```python
from build123d import *

# Parameters (mm, degrees)
SKETCH1_W           = 70
SKETCH1_H           = 55
BOSS_EXTRUDE1_DEPTH = 2
SKETCH2_W           = 73.35025282
SKETCH2_H           = 59
BOSS_EXTRUDE3_DEPTH = 2
BOSS_EXTRUDE4_DEPTH = 28
BOSS_EXTRUDE5_DEPTH = 34
SKETCH7_W           = 3
SKETCH7_H           = 23
CUT_EXTRUDE1_DEPTH  = 11
SKETCH9_R           = 1.4
CUT_EXTRUDE2_DEPTH  = 11
SKETCH10_W          = 8
SKETCH10_H          = 10
BOSS_EXTRUDE6_DEPTH = 5
CUT_EXTRUDE3_REACH  = 35.573
SKETCH12_W          = 13
SKETCH12_H          = 2
BOSS_EXTRUDE7_DEPTH = 6
SKETCH13_R          = 1.45
CUT_EXTRUDE4_DEPTH  = 10
BOSS_EXTRUDE8_DEPTH = 10
SKETCH15_R          = 1.4
CUT_EXTRUDE5_DEPTH  = 10


with BuildPart() as part:
    # Sketch1 → Boss-Extrude1 (new body)
    with BuildSketch(Plane(origin=(0, 0, 0), x_dir=(1, 0, 0), z_dir=(0, 1, 0))):
        with Locations((35, -27.5)):
            Rectangle(SKETCH1_W, SKETCH1_H)
    extrude(amount=BOSS_EXTRUDE1_DEPTH)

    # Sketch2 → Boss-Extrude3 (add)
    with BuildSketch(Plane(origin=(0, 0, 0), x_dir=(1, 0, 0), z_dir=(0, 1, 0))):
        with Locations((35.32487359, -27.5)):
            Rectangle(SKETCH2_W, SKETCH2_H)
    extrude(amount=BOSS_EXTRUDE3_DEPTH)

    # Sketch3 → Boss-Extrude4 (add)
    with BuildSketch(Plane(origin=(0, 2, 0), x_dir=(1, 0, 0), z_dir=(0, 1, 0))):
        Polygon((-1.35025282, 2), (72, 2), (72, -57), (-1.35025282, -57), (-1.35025282, -55), (70, -55), (70, 0), (-1.35025282, 0), align=None)
    extrude(amount=BOSS_EXTRUDE4_DEPTH)

    # Sketch5 → Boss-Extrude5 (add)
    with BuildSketch(Plane(origin=(0, 2, 0), x_dir=(1, 0, 0), z_dir=(0, 1, 0))):
        Polygon((11.64974718, 0), (8.64974718, 0), (8.64974718, -4.927247976), (8.64974718, -49.926173774), (8.64974718, -55), (11.64974718, -55), align=None)
        Polygon((8.64974718, -4.927247976), (8.64974718, 0), (3.64974718, 0), align=None)
        Polygon((8.64974718, -55), (8.64974718, -49.926173774), (3.64974718, -55), align=None)
    extrude(amount=BOSS_EXTRUDE5_DEPTH)

    # Sketch7 → Cut-Extrude1 (cut)
    with BuildSketch(Plane(origin=(0, 36, 0), x_dir=(1, 0, 0), z_dir=(0, 1, 0))):
        with Locations((10.14974718, -27.426710875)):
            Rectangle(SKETCH7_W, SKETCH7_H)
    extrude(amount=-CUT_EXTRUDE1_DEPTH, mode=Mode.SUBTRACT)

    # Sketch9 → Cut-Extrude2 (cut)
    with BuildSketch(Plane.ZY.offset(-8.64974718)):
        with Locations((13.426710875, 31)):
            Circle(SKETCH9_R)
        with Locations((41.426710875, 31)):
            Circle(SKETCH9_R)
    extrude(amount=-CUT_EXTRUDE2_DEPTH, mode=Mode.SUBTRACT)

    # Sketch10 → Boss-Extrude6 (add)
    with BuildSketch(Plane.ZY.offset(-8.64974718)):
        with Locations((27.426710875, 20)):
            Rectangle(SKETCH10_W, SKETCH10_H)
    extrude(amount=BOSS_EXTRUDE6_DEPTH)

    # Sketch11 → Cut-Extrude3 (cut, up to next)
    with BuildSketch(Plane(origin=(0, 0, 23.426710875), x_dir=(-1, 0, 0), z_dir=(0, 0, -1)), mode=Mode.PRIVATE) as cut_extrude3_sk1:
        Polygon((-8.64974718, 15), (-3.64974718, 25), (-3.64974718, 15), align=None)
    cut_extrude3_tool1 = extrude(cut_extrude3_sk1.sketch, amount=-CUT_EXTRUDE3_REACH, mode=Mode.PRIVATE) & part.part
    add(cut_extrude3_tool1.solids().sort_by_distance((5.316414, 18.333333, 23.426711))[0], mode=Mode.SUBTRACT)

    # Sketch12 → Boss-Extrude7 (add)
    with BuildSketch(Plane(origin=(0, 30, 0), x_dir=(1, 0, 0), z_dir=(0, 1, 0))):
        with Locations((5.14974718, 1)):
            Rectangle(SKETCH12_W, SKETCH12_H)
        with Locations((5.14974718, -56)):
            Rectangle(SKETCH12_W, SKETCH12_H)
    extrude(amount=BOSS_EXTRUDE7_DEPTH)

    # Sketch13 → Cut-Extrude4 (cut)
    with BuildSketch(Plane(origin=(0, 36, 0), x_dir=(1, 0, 0), z_dir=(0, 1, 0))):
        with Locations((8.61107216, -0.677247976)):
            Circle(SKETCH13_R)
        with Locations((8.673474118, -54.176173774)):
            Circle(SKETCH13_R)
    extrude(amount=-CUT_EXTRUDE4_DEPTH, mode=Mode.SUBTRACT)

    # Sketch14 → Boss-Extrude8 (add)
    with BuildSketch(Plane.ZY.offset(1.35025282)):
        Polygon((-2, 0), (-4, 4), (-4, 7), (-2, 11), align=None)
        Polygon((57, 0), (57, 11), (59, 7), (59, 4), align=None)
    extrude(amount=-BOSS_EXTRUDE8_DEPTH)

    # Sketch15 → Cut-Extrude5 (cut)
    with BuildSketch(Plane.ZY.offset(1.35025282)):
        with Locations((-2, 5.25)):
            Circle(SKETCH15_R)
        with Locations((57, 5.25)):
            Circle(SKETCH15_R)
    extrude(amount=-CUT_EXTRUDE5_DEPTH, mode=Mode.SUBTRACT)


solid = part.part
```
Here's how the part is built. I have some questions about the finished solid (model axes, mm). A direction names the side the tool comes from. Coordinates: 2 decimals unless noted, no trailing zeros. Loops run counter-clockwise (first coordinate to the right, second up) from the corner with the lowest first, then second, coordinate; pieces in that order, holes last. Notation, with made-up numbers: (-27.75, 14) - (19.25, 14) arc R14 ccw to (19.25, 29) - close; hole circle Ø8 at (56.5, 59). An arc over 180 degrees is marked (long way). Return JSON: item names as keys, results as strings. Group by question number.
Item 1: I need wall thicknesses on line 1 (Z direction, x = 31.5, y = 24.5); line 2 (X direction, y = 5, z = 25); line 3 (Y direction, x = 6.5, z = 51.5). Which ranges of each line are inside material? Lowest first, please. Write a range as from..to.
Item 2: If we section it at C-C on y = 31: Write out the boundary of the cut face in (x, z), and give its area (3 significant figures).
Item 3: If we section it at D-D on z = 30: Write out the boundary of the cut face in (x, y), and give its area (3 significant figures).
Item 4: If we section it at B-B on x = 5.5: Write out the boundary of the cut face in (y, z), and give its area (3 significant figures).
Item 5: On a 3-axis mill with a long thin cutter (end or side, diameter ignored), from which of +Z, -Z, +X, -X, +Y, -Y can I reach the whole of each face in a straight line? I mean faces 1 (the face through (41, 16, 0)), 2 (the face through (6.2, 19.9, 27.4)), 3 (the face through (4, 9, -3)), 4 (the face through (4, 2, 58)), 5 (the face through (10, 31, 15.927)). Say none if no direction works.
Item 6: We'd pull the mould along Y, two halves only. Please class faces 6 (the face through (3.58, 5.671, 58.335)), 7 (the face through (11.65, 19, 28)), 8 (the face through (3.58, 5.671, -0.665)), 9 (the face through (71, 30, 27)): +Y half, -Y half, draft (parallel to the pull), parting line (faces both ways), or undercut.
Item 7: Will these pins go through, and if not, where does the flat tip stop? P1, Ø4, axis at y = 27.5, z = 6.5, coming from the -X side; P2, Ø4, axis at x = 6, z = 31.5, coming from the +Y side; P3, Ø1.7, axis at y = 31, z = 41.43, coming from the +X side; P4, Ø1.5, axis at x = 9.5, y = 29.5, coming from the +Z side.
Item 8: If we section it at A-A on y = 5.25: Write out the boundary of the cut face in (x, z), and give its area (3 significant figures).
Calculated:
{
 "1": {"line 1": "z = -2..0, 55..57", "line 2": "x = 8.65..11.65, 70..72", "line 3": "y = 0..2"},
 "2": {"outline": "(-1.35, -2) - (11.65, -2) - (11.65, 12.03) - (8.65, 12.03) - (8.65, 4.93) - (3.65, 0) - (-1.35, 0) - close; (-1.35, 55) - (3.65, 55) - (8.65, 49.93) - (8.65, 42.83) - (11.65, 42.83) - (11.65, 57) - (-1.35, 57) - close; (8.65, 14.83) - (11.65, 14.83) - (11.65, 15.93) - (8.65, 15.93) - close; (8.65, 38.93) - (11.65, 38.93) - (11.65, 40.03) - (8.65, 40.03) - close; hole circle Ø2.9 at (8.61, 0.68); hole circle Ø2.9 at (8.67, 54.18)", "area": "143 mm^2"},
 "3": {"outline": "(-1.35, 0) - (72, 0) - (72, 30) - (70, 30) - (70, 2) - (11.65, 2) - (11.65, 25) - (3.65, 25) - (8.65, 15) - (8.65, 2) - (-1.35, 2) - close", "area": "297 mm^2"},
 "4": {"outline": "(0, -2) - (4, -4) - (7, -4) - (11, -2) - (36, -2) - (36, 1.82) - (2, 1.82) - (2, 53.12) - (36, 53.12) - (36, 57) - (11, 57) - (7, 59) - (4, 59) - (0, 57) - close; (21.3, 23.43) - (25, 23.43) - (25, 31.43) - (21.3, 31.43) - close; hole circle Ø2.8 at (5.25, -2); hole circle Ø2.8 at (5.25, 57)", "area": "425 mm^2"},
 "5": {"face 1": "+Y", "face 2": "-X", "face 3": "-Z, +X, -X, +Y", "face 4": "+Z, +X, -X, -Y", "face 5": "-X, +Y"},
 "6": {"face 6": "undercut", "face 7": "draft", "face 8": "undercut", "face 9": "+Y half"},
 "7": {"P1": "stops at x = 8.22", "P2": "stops at y = 25", "P3": "passes through", "P4": "stops at z = 57"},
 "8": {"outline": "(-1.35, -4) - (8.65, -4) - (8.65, -3.4) - (-1.35, -3.4) - close; (-1.35, -0.6) - (8.65, -0.6) - (8.65, -2) - (72, -2) - (72, 57) - (8.65, 57) - (8.65, 55.6) - (-1.35, 55.6) - (-1.35, 55) - (3.65, 55) - (8.65, 49.93) - (8.65, 4.93) - (3.65, 0) - (-1.35, 0) - close; (-1.35, 58.4) - (8.65, 58.4) - (8.65, 59) - (-1.35, 59) - close; hole (11.65, 0) - (70, 0) - (70, 55) - (11.65, 55) - close", "area": "577 mm^2"}
}
